Geometry: final body of the model. Coordinates: model frame, mm. A direction names the side the tool comes from. Round coordinates to 2 decimals unless told otherwise and drop trailing zeros. Write each question's results on one line, items separated by ' | '.
Autodesk Inventor part; units mm, degrees
ref_plane "YZ Plane" through (0, 0, 0) normal (1, 0, 0) x (0, 1, 0)
ref_plane "XZ Plane" through (0, 0, 0) normal (0, 1, 0) x (-1, 0, 0)
ref_plane "XY Plane" through (0, 0, 0) normal (0, 0, 1) x (1, 0, 0)
sketch "Sketch1" plane through (0, 0, 0) normal (0, 1, 0) x (-1, 0, 0)
  circle A0 centre (0, 0) radius 101.6
  line L0 (101.6, -101.6) -> (101.6, 533.4)
  line L1 (101.6, 533.4) -> (-609.6, 533.4)
  line L2 (-609.6, 533.4) -> (-609.6, -101.6)
  line L3 (-609.6, -101.6) -> (101.6, -101.6)
  arc A1 (0, 381) -> (-381, 0) centre (0, 0) ccw
  line L4 (-482.6, 12.7) -> (-482.6, -101.6)
  line L5 (-381, -101.6) -> (-381, 0)
  arc A2 (0, 393.7) -> (-393.7, 0) centre (0, 0) ccw
  line L6 (-393.7, 0) -> (-393.7, -101.6)
  line L7 (0, 393.7) -> (101.6, 393.7)
  line L8 (0, 381) -> (101.6, 381)
  dimension "d0" = 203.2
  dimension "d2" = 711.2
  dimension "d5" = 279.4
  dimension "d93" = 12.7
  dimension "d104" = 635
extrude "Extrusion1" add sketch "Sketch1" along normal blind 63.5 contours L8 A1 L5 L3 L6 A2 L7 L0
sketch "Sketch5" plane through (0, 63.5, 0) normal (0, 1, 0) x (1, 0, 0)
  line L0 (393.7, 0) -> (393.7, 101.6)
  line L1 (393.7, 101.6) -> (381, 101.6)
  line L2 (381, 101.6) -> (381, 0)
  arc A0 (0, -381) -> (381, 0) centre (0, 0) ccw
  line L3 (0, -381) -> (-101.6, -381)
  line L4 (-101.6, -381) -> (-101.6, -393.7)
  circle A1 centre (-95.25, -387.35) radius 3.3782
  circle A2 centre (0, -387.35) radius 3.3782
  circle A3 centre (387.35, 0) radius 3.3782
  circle A4 centre (387.35, 95.25) radius 3.3782
  circle A5 centre (387.35, 83.3438) radius 3.3782
  circle A6 centre (387.35, 71.4375) radius 3.3782
  circle A7 centre (387.35, 59.5313) radius 3.3782
  circle A8 centre (387.35, 47.625) radius 3.3782
  circle A9 centre (387.35, 35.7188) radius 3.3782
  circle A10 centre (387.35, 23.8125) radius 3.3782
  circle A11 centre (387.35, 11.9063) radius 3.3782
  circle A12 centre (-85.725, -387.35) radius 3.3782
  circle A13 centre (-76.2, -387.35) radius 3.3782
  circle A14 centre (-66.675, -387.35) radius 3.3782
  circle A15 centre (-57.15, -387.35) radius 3.3782
  circle A16 centre (-47.625, -387.35) radius 3.3782
  circle A17 centre (-38.1, -387.35) radius 3.3782
  circle A18 centre (-28.575, -387.35) radius 3.3782
  circle A19 centre (-19.05, -387.35) radius 3.3782
  circle A20 centre (-9.525, -387.35) radius 3.3782
  circle A21 centre (10.3115, -387.2127) radius 3.3782
  circle A22 centre (20.6156, -386.801) radius 3.3782
  circle A23 centre (30.9051, -386.1151) radius 3.3782
  circle A24 centre (41.1728, -385.1556) radius 3.3782
  circle A25 centre (51.4112, -383.923) radius 3.3782
  circle A26 centre (61.6132, -382.4184) radius 3.3782
  circle A27 centre (71.7716, -380.6427) radius 3.3782
  circle A28 centre (81.8791, -378.5972) radius 3.3782
  circle A29 centre (91.9285, -376.2834) radius 3.3782
  circle A30 centre (101.9128, -373.7028) radius 3.3782
  circle A31 centre (111.8248, -370.8574) radius 3.3782
  circle A32 centre (121.6576, -367.7492) radius 3.3782
  circle A33 centre (131.4042, -364.3802) radius 3.3782
  circle A34 centre (141.0576, -360.7531) radius 3.3782
  circle A35 centre (150.611, -356.8702) radius 3.3782
  circle A36 centre (160.0577, -352.7344) radius 3.3782
  circle A37 centre (169.391, -348.3486) radius 3.3782
  circle A38 centre (178.6042, -343.7158) radius 3.3782
  circle A39 centre (187.6908, -338.8395) radius 3.3782
  circle A40 centre (196.6443, -333.723) radius 3.3782
  circle A41 centre (205.4585, -328.3699) radius 3.3782
  circle A42 centre (214.1271, -322.7841) radius 3.3782
  circle A43 centre (222.6439, -316.9696) radius 3.3782
  circle A44 centre (231.0029, -310.9304) radius 3.3782
  circle A45 centre (239.1982, -304.6707) radius 3.3782
  circle A46 centre (247.2239, -298.1952) radius 3.3782
  circle A47 centre (255.0744, -291.5083) radius 3.3782
  circle A48 centre (262.7441, -284.6148) radius 3.3782
  circle A49 centre (270.2276, -277.5195) radius 3.3782
  circle A50 centre (277.5195, -270.2276) radius 3.3782
  circle A51 centre (284.6148, -262.7441) radius 3.3782
  circle A52 centre (291.5083, -255.0744) radius 3.3782
  circle A53 centre (298.1952, -247.2239) radius 3.3782
  circle A54 centre (304.6707, -239.1982) radius 3.3782
  circle A55 centre (310.9304, -231.0029) radius 3.3782
  circle A56 centre (316.9696, -222.6439) radius 3.3782
  circle A57 centre (322.7841, -214.1271) radius 3.3782
  circle A58 centre (328.3699, -205.4585) radius 3.3782
  circle A59 centre (333.723, -196.6443) radius 3.3782
  circle A60 centre (338.8395, -187.6908) radius 3.3782
  circle A61 centre (343.7158, -178.6042) radius 3.3782
  circle A62 centre (348.3486, -169.391) radius 3.3782
  circle A63 centre (352.7344, -160.0577) radius 3.3782
  circle A64 centre (356.8702, -150.611) radius 3.3782
  circle A65 centre (360.7531, -141.0576) radius 3.3782
  circle A66 centre (364.3802, -131.4042) radius 3.3782
  circle A67 centre (367.7492, -121.6576) radius 3.3782
  circle A68 centre (370.8574, -111.8248) radius 3.3782
  circle A69 centre (373.7028, -101.9128) radius 3.3782
  circle A70 centre (376.2834, -91.9285) radius 3.3782
  circle A71 centre (378.5972, -81.8791) radius 3.3782
  circle A72 centre (380.6427, -71.7716) radius 3.3782
  circle A73 centre (382.4184, -61.6132) radius 3.3782
  circle A74 centre (383.923, -51.4112) radius 3.3782
  circle A75 centre (385.1556, -41.1728) radius 3.3782
  circle A76 centre (386.1151, -30.9051) radius 3.3782
  circle A77 centre (386.801, -20.6156) radius 3.3782
  circle A78 centre (387.2127, -10.3115) radius 3.3782
  circle A79 centre (387.35, 0) radius 3.3782
  dimension "d94" = 6.7564
  dimension "d95" = 6.35
  dimension "d96" = 6.7564
  dimension "d97" = 6.7564
  dimension "d98" = 6.35
  dimension "d99" = 6.35
  dimension "d100" = 6.35
  dimension "d101" = 6.35
  dimension "d102" = 6.35
  dimension "d103" = 101.6
  dimension "d105" = 101.6
  dimension "d108" = 11.9062
  dimension "d115" = 9.525
  dimension "d122" = 90
extrude "Extrusion5" cut sketch "Sketch5" against normal blind 63.5
sketch "Sketch11" plane through (0, 63.5, 0) normal (0, 1, 0) x (1, 0, 0)
  circle A0 centre (-19.05, -387.35) radius 3.3782
  circle A1 centre (-38.1, -387.35) radius 3.3782
  circle A2 centre (-57.15, -387.35) radius 3.3782
  circle A3 centre (-76.2, -387.35) radius 3.3782
  circle A4 centre (-95.25, -387.35) radius 3.3782
  circle A5 centre (-85.725, -387.35) radius 3.3782
  circle A6 centre (-66.675, -387.35) radius 3.3782
  circle A7 centre (-47.625, -387.35) radius 3.3782
  circle A8 centre (-28.575, -387.35) radius 3.3782
  line L0 (0, -381) -> (-101.6, -381)
  line L1 (-101.6, -381) -> (-101.6, -393.7)
  line L2 (-101.6, -393.7) -> (0, -393.7)
  line L3 (-6.35, -381) -> (-6.35, -393.7)
  dimension "d142" = 95.25
extrude "Extrusion9" cut sketch "Sketch11" against normal blind 2540
equation "\"d89\" = d46"
properties part number "Outer Rail v1" material "Polycarbonate, Clear"
1. Section A-A (y = 37.5). Count the separate pieces of the cut face and the enclosed holes in it, then the cut area to 3 significant figures.
Answer key:
separate pieces: 1 | enclosed holes: 68 | area: 6,660 mm²
2. Pin query (flat end, axial travel): P1, Ø3, axis at x = 135, y = 16.5, coming from the +Z side; P2, Ø1.5, axis at x = 335.5, y = 44, coming from the -Z side; P3, Ø6, axis at x = 169.39, z = 348.35, coming from the -Y side; P4, Ø3, axis at y = 23.5, z = -2.5, coming from the -X side. Return the tip coordinate at first contact, or that it passes through.
Answer key:
P1: stops at z = 370.37 | P2: stops at z = 179.16 | P3: passes through | P4: stops at x = 381
3. Access query for faces 1 (the face through (281.43, 31.31, 275.31)), 2 (the face through (381, 31, -52)). Directions: +Z, -Z, +X, -X, +Y, -Y. A direction counts if a zero-diameter tool reaches every point of the face in a straight line with its end or side. Return the directions, or none.
Answer key:
face 1: +Z, +X, +Y, -Y | face 2: -Z, -X, +Y, -Y
4. Ray query, probe 1 along X at (y, z) = (27.5, 325.5); probe 2 along X at (y, z) = (15, -95.25); probe 3 along Z at (x, y) = (263, 56). Return the intervals inside material, ascending.
Answer key:
probe 1: x = 198.02 to 203.68, 207.24 to 212.12, 216.14 to 221.47 | probe 2: x = 381 to 383.97, 390.73 to 393.7 | probe 3: z = 275.67 to 281.25, 287.98 to 292.97
